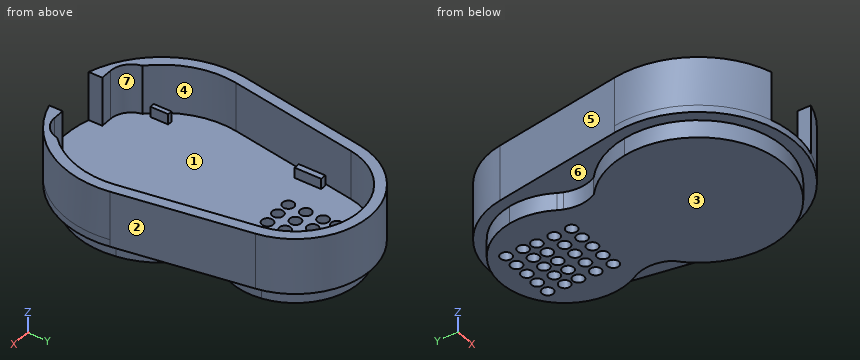
```python
from build123d import *

# Parameters (mm, degrees)
F1_DEPTH = 1
F2_DEPTH = 3.5
F4_DEPTH = 7
F3_W     = 0.8317038625
F3_H     = 3.7825570011
F3_W_2   = 0.7836289912
F3_W_3   = 0.6960576609
F3_H_2   = 2.5395583361
F3_W_4   = 0.6565612018
F5_DEPTH = 1.5
F3_R     = 0.8088750424
F6_DEPTH = 5


with BuildPart() as f1:
    # F0 (on Top) → F1 (new body)
    with BuildSketch(Plane.XY):
        with BuildLine():
            ThreePointArc((10.5534817095, 15.4336250836), (0, 24.3689653978), (-10.5534817095, 15.4336250836))
            Line((-10.5534817095, 15.4336250836), (-13.6603478203, -3.1468722986))
            ThreePointArc((-13.6603478203, -3.1468722986), (0, -19.2810346022), (13.6603478203, -3.1468722986))
            Line((13.6603478203, -3.1468722986), (10.5534817095, 15.4336250836))
        make_face()
        with BuildLine():
            ThreePointArc((-7.9318843768, 3.9042591925), (-7.9136479922, 3.9365495997), (-7.8956354366, 3.9689653978))
            ThreePointArc((-7.8956354366, 3.9689653978), (-7.2435768772, 6.1726329025), (-7.5742542147, 8.4468323957))
            ThreePointArc((-7.5742542147, 8.4468323957), (-7.7343170695, 8.8265985648), (-7.9230829656, 9.1929452547))
            ThreePointArc((-7.9230829656, 9.1929452547), (-8.9621513279, 12.0910415797), (-8.9753909866, 15.1697507381))
            ThreePointArc((-8.9753909866, 15.1697507381), (0, 22.7689653978), (8.9753909866, 15.1697507381))
            ThreePointArc((8.9753909866, 15.1697507381), (8.9621513279, 12.0910415797), (7.9230829656, 9.1929452547))
            ThreePointArc((7.9230829656, 9.1929452547), (7.7343170695, 8.8265985648), (7.5742542147, 8.4468323957))
            ThreePointArc((7.5742542147, 8.4468323957), (7.2435768772, 6.1726329025), (7.8956354366, 3.9689653978))
            ThreePointArc((7.8956354366, 3.9689653978), (7.9136479922, 3.9365495997), (7.9318843768, 3.9042591925))
            ThreePointArc((7.9318843768, 3.9042591925), (10.6545198078, 0.6141045745), (12.0822570973, -3.4107466441))
            ThreePointArc((12.0822570973, -3.4107466441), (0, -17.6810346022), (-12.0822570973, -3.4107466441))
            ThreePointArc((-12.0822570973, -3.4107466441), (-10.6545198078, 0.6141045745), (-7.9318843768, 3.9042591925))
        make_face(mode=Mode.SUBTRACT)
        with BuildLine():
            Line((7.8956354366, 3.9689653978), (-7.8956354366, 3.9689653978))
            ThreePointArc((-7.8956354366, 3.9689653978), (-7.9136479922, 3.9365495997), (-7.9318843768, 3.9042591925))
            ThreePointArc((-7.9318843768, 3.9042591925), (-10.6545198078, 0.6141045745), (-12.0822570973, -3.4107466441))
            ThreePointArc((-12.0822570973, -3.4107466441), (0, -17.6810346022), (12.0822570973, -3.4107466441))
            ThreePointArc((12.0822570973, -3.4107466441), (10.6545198078, 0.6141045745), (7.9318843768, 3.9042591925))
            ThreePointArc((7.9318843768, 3.9042591925), (7.9136479922, 3.9365495997), (7.8956354366, 3.9689653978))
        make_face()
        with BuildLine():
            ThreePointArc((-7.9230829656, 9.1929452547), (-7.7343170695, 8.8265985648), (-7.5742542147, 8.4468323957))
            ThreePointArc((-7.5742542147, 8.4468323957), (0, 4.4689653978), (7.5742542147, 8.4468323957))
            ThreePointArc((7.5742542147, 8.4468323957), (7.7343170695, 8.8265985648), (7.9230829656, 9.1929452547))
            ThreePointArc((7.9230829656, 9.1929452547), (8.9621513279, 12.0910415797), (8.9753909866, 15.1697507381))
            ThreePointArc((8.9753909866, 15.1697507381), (0, 22.7689653978), (-8.9753909866, 15.1697507381))
            ThreePointArc((-8.9753909866, 15.1697507381), (-8.9621513279, 12.0910415797), (-7.9230829656, 9.1929452547))
        make_face()
        with BuildLine():
            ThreePointArc((-7.5742542147, 8.4468323957), (-7.2435768772, 6.1726329025), (-7.8956354366, 3.9689653978))
            Line((-7.8956354366, 3.9689653978), (7.8956354366, 3.9689653978))
            ThreePointArc((7.8956354366, 3.9689653978), (7.2435768772, 6.1726329025), (7.5742542147, 8.4468323957))
            ThreePointArc((7.5742542147, 8.4468323957), (0, 4.4689653978), (-7.5742542147, 8.4468323957))
        make_face()
    extrude(amount=-F1_DEPTH)

    # F0 (on Top) → F2 (join)
    with BuildSketch(Plane.XY):
        with BuildLine():
            ThreePointArc((-7.5742542147, 8.4468323957), (-7.2435768772, 6.1726329025), (-7.8956354366, 3.9689653978))
            Line((-7.8956354366, 3.9689653978), (7.8956354366, 3.9689653978))
            ThreePointArc((7.8956354366, 3.9689653978), (7.2435768772, 6.1726329025), (7.5742542147, 8.4468323957))
            ThreePointArc((7.5742542147, 8.4468323957), (0, 4.4689653978), (-7.5742542147, 8.4468323957))
        make_face()
        with BuildLine():
            Line((7.8956354366, 3.9689653978), (-7.8956354366, 3.9689653978))
            ThreePointArc((-7.8956354366, 3.9689653978), (-7.9136479922, 3.9365495997), (-7.9318843768, 3.9042591925))
            ThreePointArc((-7.9318843768, 3.9042591925), (-10.6545198078, 0.6141045745), (-12.0822570973, -3.4107466441))
            ThreePointArc((-12.0822570973, -3.4107466441), (0, -17.6810346022), (12.0822570973, -3.4107466441))
            ThreePointArc((12.0822570973, -3.4107466441), (10.6545198078, 0.6141045745), (7.9318843768, 3.9042591925))
            ThreePointArc((7.9318843768, 3.9042591925), (7.9136479922, 3.9365495997), (7.8956354366, 3.9689653978))
        make_face()
        with BuildLine():
            ThreePointArc((-7.9230829656, 9.1929452547), (-7.7343170695, 8.8265985648), (-7.5742542147, 8.4468323957))
            ThreePointArc((-7.5742542147, 8.4468323957), (0, 4.4689653978), (7.5742542147, 8.4468323957))
            ThreePointArc((7.5742542147, 8.4468323957), (7.7343170695, 8.8265985648), (7.9230829656, 9.1929452547))
            ThreePointArc((7.9230829656, 9.1929452547), (8.9621513279, 12.0910415797), (8.9753909866, 15.1697507381))
            ThreePointArc((8.9753909866, 15.1697507381), (0, 22.7689653978), (-8.9753909866, 15.1697507381))
            ThreePointArc((-8.9753909866, 15.1697507381), (-8.9621513279, 12.0910415797), (-7.9230829656, 9.1929452547))
        make_face()
    extrude(amount=-F2_DEPTH)

    # F3 (on face) → F4 (join)
    with BuildSketch(Plane.XY):
        with BuildLine():
            Line((-4, -16.7553447357), (-5.65, -16.7553447357))
            ThreePointArc((-5.65, -16.7553447357), (-7.5717587133, -16.0590034448), (-8.6013841311, -14.2932403677))
            ThreePointArc((-8.6013841311, -14.2932403677), (-11.7334001707, -9.284581077), (-12.1808877675, -3.3942544975))
            Line((-12.1808877675, -3.3942544975), (-9.0740216568, 15.1862428847))
            ThreePointArc((-9.0740216568, 15.1862428847), (0, 22.8689653978), (9.0740216568, 15.1862428847))
            Line((9.0740216568, 15.1862428847), (12.1808877675, -3.3942544975))
            ThreePointArc((12.1808877675, -3.3942544975), (11.7334001707, -9.284581077), (8.6013841311, -14.2932403677))
            ThreePointArc((8.6013841311, -14.2932403677), (7.5717587133, -16.0590034448), (5.65, -16.7553447357))
            Line((5.65, -16.7553447357), (4, -16.7553447357))
            Line((4, -16.7553447357), (4, -17.9553447357))
            Line((4, -17.9553447357), (4, -18.6908422931))
            ThreePointArc((4, -18.6908422931), (11.7633210481, -12.7417649295), (13.6603478203, -3.1468722986))
            Line((13.6603478203, -3.1468722986), (10.5534817095, 15.4336250836))
            ThreePointArc((10.5534817095, 15.4336250836), (0, 24.3689653978), (-10.5534817095, 15.4336250836))
            Line((-10.5534817095, 15.4336250836), (-13.6603478203, -3.1468722986))
            ThreePointArc((-13.6603478203, -3.1468722986), (-11.7633210481, -12.7417649295), (-4, -18.6908422931))
            Line((-4, -18.6908422931), (-4, -17.9553447357))
            Line((-4, -17.9553447357), (-4, -16.7553447357))
        make_face()
    extrude(amount=F4_DEPTH)

    # F3 (on face) → F5 (join)
    with BuildSketch(Plane.XY):
        with Locations((-9.0658519313, 9.3533767637)):
            Rectangle(F3_W, F3_H)
        with Locations((9.0418144956, 9.3533767637)):
            Rectangle(F3_W_2, F3_H)
        with Locations((8.9980288304, -11.8910893798)):
            Rectangle(F3_W_3, F3_H_2)
        with Locations((-8.9782806009, -11.8910893798)):
            Rectangle(F3_W_4, F3_H_2)
    extrude(amount=F5_DEPTH)

    # F3 (on face) → F6 (cut)
    with BuildSketch(Plane.XY):
        with Locations((-3.9931656793, 19.2196834832)):
            Circle(F3_R)
        with Locations((-1.8931656793, 19.2196834832)):
            Circle(F3_R)
        with Locations((0.2068343207, 19.2196834832)):
            Circle(F3_R)
        with Locations((2.3068343207, 19.2196834832)):
            Circle(F3_R)
        with Locations((4.4068343207, 19.2196834832)):
            Circle(F3_R)
        with Locations((4.4068343207, 16.7862419039)):
            Circle(F3_R)
        with Locations((2.3068343207, 16.7862419039)):
            Circle(F3_R)
        with Locations((0.2068343207, 16.7862419039)):
            Circle(F3_R)
        with Locations((-1.8931656793, 16.7862419039)):
            Circle(F3_R)
        with Locations((-3.9931656793, 16.7862419039)):
            Circle(F3_R)
        with Locations((-3.9502955042, 14.8469135165)):
            Circle(F3_R)
        with Locations((-1.8502955042, 14.8469135165)):
            Circle(F3_R)
        with Locations((0.2497044958, 14.8469135165)):
            Circle(F3_R)
        with Locations((2.3497044958, 14.8469135165)):
            Circle(F3_R)
        with Locations((4.4497044958, 14.8469135165)):
            Circle(F3_R)
        with Locations((-3.9502955042, 12.3752485961)):
            Circle(F3_R)
        with Locations((-1.8502955042, 12.3752485961)):
            Circle(F3_R)
        with Locations((0.2497044958, 12.3752485961)):
            Circle(F3_R)
        with Locations((2.3497044958, 12.3752485961)):
            Circle(F3_R)
        with Locations((4.4497044958, 12.3752485961)):
            Circle(F3_R)
        with Locations((-3.9502955042, 9.8736844957)):
            Circle(F3_R)
        with Locations((-1.8502955042, 9.8736844957)):
            Circle(F3_R)
        with Locations((0.2497044958, 9.8736844957)):
            Circle(F3_R)
        with Locations((2.3497044958, 9.8736844957)):
            Circle(F3_R)
        with Locations((4.4497044958, 9.8736844957)):
            Circle(F3_R)
    extrude(amount=-F6_DEPTH, mode=Mode.SUBTRACT)


solid = f1.part
```
Could you check a few things on this model? Use its own coordinates, in mm. Face numbers are marked on the shaded views. A direction names the side the tool comes from. Give positions to 0.01 mm unless a question says otherwise; leave off trailing zeros. Write each loop counter-clockwise with the first axis right and the second up, starting at its lowest first coordinate (ties: lowest second). Pieces come first, ordered by that corner, then holes. Notation, with made-up numbers: (79.5, 52) - (106.5, 52) arc R19 cw to (106.5, 68) - close; hole circle Ø4 at (18, 72). An arc over 180 degrees is marked (long way). One line per item, written item: value. Start each with the question number.
Item 1: Imagine slicing it at A-A, the plane x = 0. Give the number of separate pieces and of enclosed holes in the cut face, and give its area (3 significant figures).
Item 2: Please list where these lines run through material, in increasing order: line 1 (X direction, y = -5, z = 2); line 2 (Y direction, x = 2, z = -0.25); line 3 (Z direction, x = -9.5, y = 0). Write a range as from..to.
Item 3: Imagine slicing it at D-D, the plane x = -10. List the corners of the cut face in (y, z) for me, and give its area (3 significant figures).
Item 4: Imagine slicing it at B-B, the plane z = 5.75. List the corners of the cut face in (x, y) for me.
Item 5: Imagine slicing it at C-C, the plane y = 1. List the corners of the cut face in (x, z) for me, and give its area (3 significant figures).
Item 6: If we mould it in two halves opening along Y, with no side actions, what happens to the marked faces 1, 2, 3 and 4? For each: +Y half, -Y half, draft (parallel to the pull), parting line (faces both ways), or undercut.
Item 7: Which directions (+Z, -Z, +X, -X, +Y, -Y) give clear straight access to the entire face, cutting with the end or side of a thin tool? Please do the marked faces 5, 6 and 7.
Item 8: I'm going to push flat-ended pins straight in: pin 1 (6 mm diameter, centred on x = 11, z = 2, fed in from -Y); pin 2 (0.9 mm diameter, centred on x = -9, y = 9.5, fed in from +Z); pin 3 (2.5 mm diameter, centred on x = -1.85, y = 9.87, fed in from -Z); pin 4 (1.2 mm diameter, centred on y = 8.5, z = 1, fed in from +X). Where does each tip first touch, or does it pass through?
Geometry says:
1. separate pieces: 6
1. enclosed holes: 0
1. area: 128 mm^2
2. line 1: -13.84..-12.34, 12.34..13.84
2. line 2: -19.14..9.14, 10.6..11.65, 13.1..14.12, 15.58..16.04, 17.53..18.47, 19.97..24.18
2. line 3: -3.5..0
3. outline: (-15.01, -1) - (-12.51, -1) - (-12.51, -3.5) - (1.64, -3.5) - (1.64, -1) - (17.48, -1) - (17.48, 7) - (9.65, 7) - (9.65, 0) - (-12.68, 0) - (-12.68, 7) - (-15.01, 7) - close
3. area: 139 mm^2
4. outline: (-13.66, -3.15) arc R13.85 ccw to (-4, -18.69) - (-4, -16.76) - (-5.65, -16.76) arc R3 cw to (-8.6, -14.29) arc R12.35 cw to (-12.18, -3.39) - (-9.07, 15.19) arc R9.2 cw to (9.07, 15.19) - (12.18, -3.39) arc R12.35 cw to (8.6, -14.29) arc R3 cw to (5.65, -16.76) - (4, -16.76) - (4, -18.69) arc R13.85 ccw to (13.66, -3.15) - (10.55, 15.43) arc R10.7 ccw to (-10.55, 15.43) - close
5. outline: (-12.97, -1) - (-10.43, -1) - (-10.43, -3.5) - (10.43, -3.5) - (10.43, -1) - (12.97, -1) - (12.97, 7) - (11.45, 7) - (11.45, 0) - (-11.45, 0) - (-11.45, 7) - (-12.97, 7) - close
5. area: 99.4 mm^2
6. face 1: undercut
6. face 2: +Y half
6. face 3: draft
6. face 4: undercut
7. face 5: +Z, -Z, -X, +Y
7. face 6: -Z
7. face 7: +Z
8. pin 1: y = -16.74
8. pin 2: z = 1.5
8. pin 3: z = -3.5
8. pin 4: x = 11.81
